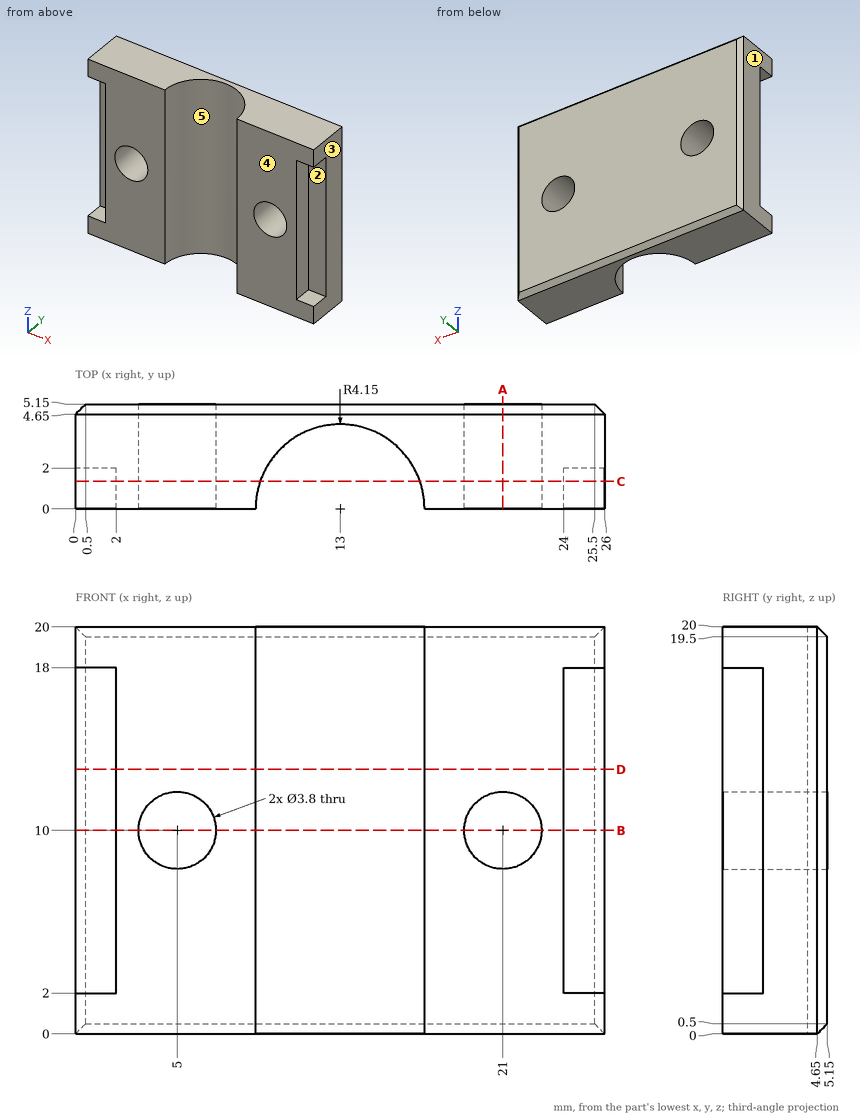
For this review, use the dimensioned drawing (mm, ordinates from the lowest corner) and the shaded views. A direction names the side the tool comes from. Give positions to 0.01 mm unless a question says otherwise; leave off trailing zeros. Order: outer loops, then holes, each group sorted by start corner. A loop starts at its lowest first (then second) coordinate and runs counter-clockwise, first axis right, second up.
1) Insertion check: pin 1 (1 mm diameter, centred on y = 1, z = 11, fed in from -X); pin 2 (0.6 mm diameter, centred on x = 0.5, z = 13.5, fed in from -Y); pin 3 (0.6 mm diameter, centred on y = 1, z = 9, fed in from +X). Each pin has a flat end and moves straight along its axis. Give the tip position at first contact, or say it passes through.
2) Wall thickness on line 1 (Z direction, x = 1, y = 1.8); line 2 (X direction, y = 3.15, z = 10); line 3 (X direction, y = 1.35, z = 10): over which ranges is each line inside the solid? List them lowest first.
3) Take a section at B-B (z = 10). Give the boundary of the cut face in (x, y).
4) Take a section at D-D (z = 13). Give the boundary of the cut face in (x, y), then the cut area to 3 significant figures.
5) Take a section at A-A (x = 21). Give the boundary of the cut face in (y, z).
6) For the marked faces 1 and 2, list the 3-axis set-ups (+Z, -Z, +X, -X, +Y, -Y) from which the entire face can be reached by the end or side of a thin tool; tool diameter is ignored.
7) Take a section at C-C (y = 1.35). Give the boundary of the cut face in (x, z).
8) The part is to be moulded in two halves that separate along X. For the marked faces 3, 4 and 5, say which applies: released by +X, released by -X, zero draft, split by the parting line, or undercut.
Derived:
1. pin 1: stops at x = 2
1. pin 2: stops at y = 2
1. pin 3: stops at x = 24
2. line 1: z = 0 to 2, 18 to 20
2. line 2: x = 0 to 3.1, 6.9 to 10.3, 15.7 to 19.1, 22.9 to 26
2. line 3: x = 2 to 3.1, 6.9 to 9.08, 16.92 to 19.1, 22.9 to 24
3. outline: (0, 2) - (2, 2) - (2, 0) - (3.1, 0) - (3.1, 5.15) - (0.5, 5.15) - (0, 4.65) - close; (6.9, 0) - (8.85, 0) arc R4.15 cw to (17.15, 0) - (19.1, 0) - (19.1, 5.15) - (6.9, 5.15) - close; (22.9, 0) - (24, 0) - (24, 2) - (26, 2) - (26, 4.65) - (25.5, 5.15) - (22.9, 5.15) - close
4. outline: (0, 2) - (2, 2) - (2, 0) - (8.85, 0) arc R4.15 cw to (17.15, 0) - (24, 0) - (24, 2) - (26, 2) - (26, 4.65) - (25.5, 5.15) - (0.5, 5.15) - (0, 4.65) - close
4. area: 98.6 mm2
5. outline: (0, 0) - (4.65, 0) - (5.15, 0.5) - (5.15, 8.1) - (0, 8.1) - close; (0, 11.9) - (5.15, 11.9) - (5.15, 19.5) - (4.65, 20) - (0, 20) - close
6. face 1: +Z, -Z, -X, +Y, -Y
6. face 2: +X, -Y
7. outline: (0, 0) - (9.08, 0) - (9.08, 20) - (0, 20) - (0, 18) - (2, 18) - (2, 2) - (0, 2) - close; (16.92, 0) - (26, 0) - (26, 2) - (24, 2) - (24, 18) - (26, 18) - (26, 20) - (16.92, 20) - close; hole circle Ø3.8 at (5, 10); hole circle Ø3.8 at (21, 10)
8. face 3: released by +X
8. face 4: zero draft
8. face 5: undercut
